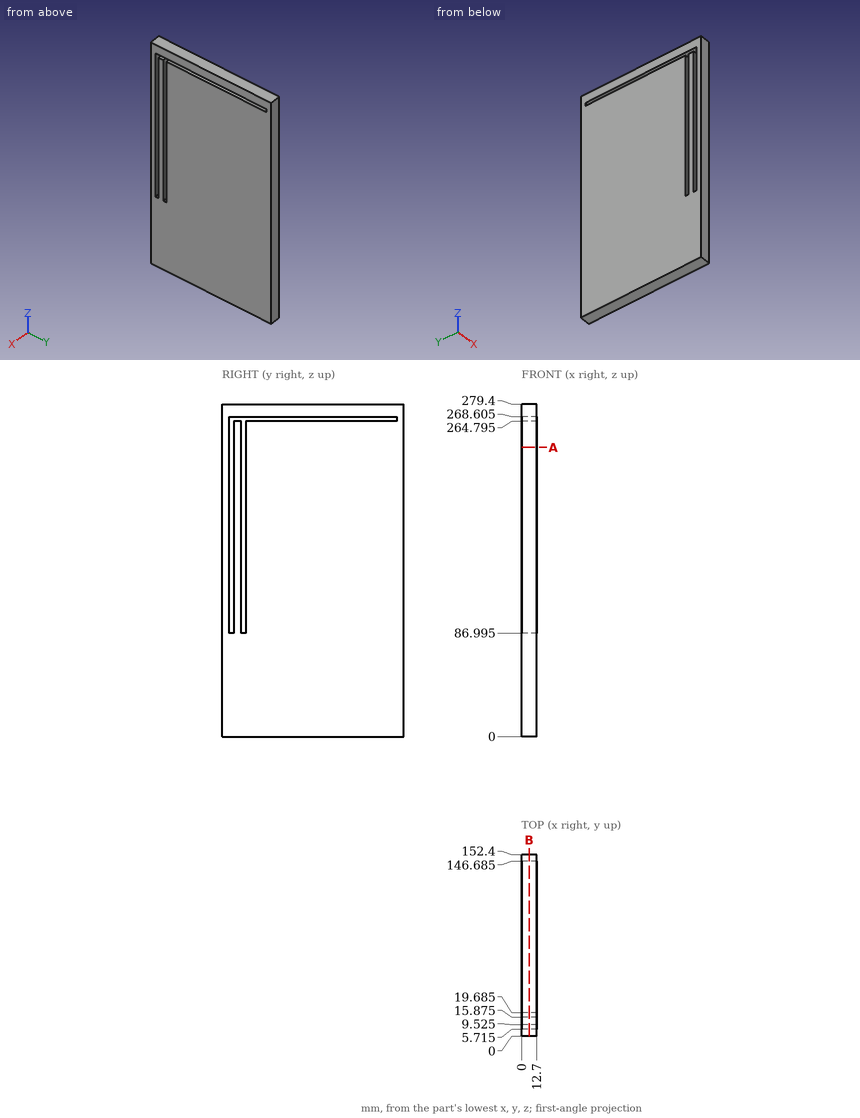
For this review, use the dimensioned drawing (mm, ordinates from the lowest corner) and the shaded views. Give positions to 0.01 mm unless a question says otherwise; leave off trailing zeros. Order: outer loops, then holes, each group sorted by start corner. A loop starts at its lowest first (then second) coordinate and runs counter-clockwise, first axis right, second up. Notation, with made-up numbers: (-21, 19) -> (32, 19) arc R24 cw to (32, 50) -> close; hole circle Ø4 at (31.25, 15.25). An arc over 180 degrees is marked (long way). Write item = value, one per line. Start each with the question number.
(1) Take a section at B-B (x = 6.25). Write out the cut boundary in (y, z) (3 decimals), plus the area to 3 significant figures.
(2) For L1, parallel to Y at x = 5.5, z = 183.5 (3 decimals); L2, parallel to Z at x = 9.75, y = 92.5 (3 decimals); L3, parallel to Z at x = 8.25, y = 6 (3 decimals), list the stretches that pass through material, from the lowest coordinate up. Write a range as from..to.
(3) Take a section at A-A (z = 243). Write out the cut boundary in (x, y) (3 decimals), plus the area to 3 significant figures.
Returned:
q1.outline = (0, 0) -> (152.4, 0) -> (152.4, 279.4) -> (0, 279.4) -> close; hole (5.715, 86.995) -> (9.525, 86.995) -> (9.525, 264.795) -> (15.875, 264.795) -> (15.875, 86.995) -> (19.685, 86.995) -> (19.685, 264.795) -> (146.685, 264.795) -> (146.685, 268.605) -> (5.715, 268.605) -> close
q1.area = 40,700 mm²
q2.L1 = 0..5.715, 9.525..15.875, 19.685..152.4
q2.L2 = 0..264.795, 268.605..279.4
q2.L3 = 0..86.995, 268.605..279.4
q3.outline = (0, 0) -> (12.7, 0) -> (12.7, 5.715) -> (0, 5.715) -> close; (0, 9.525) -> (12.7, 9.525) -> (12.7, 15.875) -> (0, 15.875) -> close; (0, 19.685) -> (12.7, 19.685) -> (12.7, 152.4) -> (0, 152.4) -> close
q3.area = 1,840 mm²
